Input: part model. Units: mm. Frame: model coordinates. A direction names the side the tool comes from. Give positions to 0.01 mm unless a question says otherwise; leave off trailing zeros. Loops run counter-clockwise (first coordinate to the right, second up) from the corner with the lowest first, then second, coordinate; pieces in that order, holes last. Notation, with made-up numbers: M 46,7 L 84,7 A15 cw 84,24 Z; hole C 42,84.25 d1. An arc over 180 degrees is marked long. One line per item, written item: value. Start each with the question number.
(1) Pin query (flat end, axial travel): P1, Ø5.5, axis at x = 6, y = 41.5, coming from the +Z side; P2, Ø1.5, axis at y = 27, z = 161.5, coming from the +X side; P3, Ø4, axis at x = -3, y = 46, coming from the -Z side. Return the tip coordinate at first contact, or that it passes through.
(2) Section D-D on z = -141. Output: boundary loops of the cut face in (x, y), plus the area to 3 significant figures.
(3) Pull-direction query (X, two-part tool) for faces 4 (the flat face through (-100.039, 54, -52)), 5 (the flat face through (-1, 38.1, 5)), 6 (the flat face through (3, 52.07, 68)), 7 (the flat face through (242.861, 22, -59)); classes: released by +X, released by -X, zero draft, split by the parting line, or undercut.
(4) Section A-A on x = 211.5. Output: boundary loops of the cut face in (y, z).
(5) Ray query, line 1 along Z through (x, y) = (94.5, 47); line 2 along Z through (x, y) = (-195, 30); line 3 along X through (y, z) = (31.5, 17). Return the intervals inside material, ascending. Write a range as from..to.
(6) Access query for faces 1 (the flat face through (-115, 24, -187.843)), 2 (the flat face through (-195, 22.86, -106)), 3 (the flat face through (-188.939, 22, 223)). Directions: +Z, -Z, +X, -X, +Y, -Y. A direction counts if a zero-diameter tool reaches every point of the face in a straight line with its end or side. Return the directions, or none.
(7) Section C-C on x = 35. Output: boundary loops of the cut face in (y, z).
(8) Section B-B on z = 120. Output: boundary loops of the cut face in (x, y).
```python
from build123d import *

# Parameters (mm, degrees)
SKETCH1_W                = 406.4
SKETCH1_H                = 406.4
SKETCH1_W_2              = 381
SKETCH1_H_2              = 381
BOSS_EXTRUDE2_DEPTH      = 38.1
SKETCH2_W                = 406.4
SKETCH2_H                = 406.4
BOSS_EXTRUDE3_DEPTH      = 5.08
CUT_EXTRUDE3_DEPTH       = 5.08
CUT_EXTRUDE4_DEPTH       = 446.859951222
CUT_EXTRUDE4_DEPTH_BACK  = 446.859951222
SKETCH6_R                = 5.08
CUT_EXTRUDE6_DEPTH       = 5.08
SKETCH8_W                = 457.2
SKETCH8_H                = 43.18
BOSS_EXTRUDE4_DEPTH      = 12.7
SKETCH9_R                = 5.08
CUT_EXTRUDE7_DEPTH       = 462.214953622
FILLET2_R                = 15.24
FILLET3_R                = 5.08
FILLET4_R                = 6.35
CUT_EXTRUDE8_DEPTH       = 473.102217157
CUT_EXTRUDE8_DEPTH_BACK  = 473.102217157
SKETCH10_W               = 25.4
SKETCH10_H               = 10.16
CUT_EXTRUDE9_DEPTH       = 316.013546928
CUT_EXTRUDE9_DEPTH_BACK  = 316.013546928
SKETCH11_W               = 10.16
SKETCH11_H               = 25.4
SKETCH13_W               = 38.1
SKETCH13_H               = 17.78
BOSS_EXTRUDE6_DEPTH      = 406.4
FILLET5_R                = 13.97
CUT_EXTRUDE10_DEPTH      = 475.059186858
CUT_EXTRUDE10_DEPTH_BACK = 101.6
SKETCH14_W               = 157.48
SKETCH14_H               = 20.829558228
SKETCH17_W               = 157.48
SKETCH17_H               = 21.78032637
CUT_EXTRUDE11_DEPTH      = 101.6
BOSS_EXTRUDE7_START      = -12.7
SKETCH18_W               = 375.92
SKETCH18_H               = 43.18
BOSS_EXTRUDE7_DEPTH      = 12.7
SKETCH19_W               = 12.7
SKETCH19_H               = 43.18
BOSS_EXTRUDE8_DEPTH      = 38.1
SKETCH20_R               = 5.08
CUT_EXTRUDE12_DEPTH      = 413.381445795
SKETCH21_W               = 23.212308842
SKETCH21_H               = 297.780762004
BOSS_EXTRUDE10_DEPTH     = 5.08
SKETCH22_W               = 25.4
SKETCH22_H               = 12.7
CUT_EXTRUDE13_DEPTH      = 500.147895153
SKETCH23_W               = 25.4
SKETCH23_H               = 12.7
CUT_EXTRUDE14_DEPTH      = 342.010118149


with BuildPart() as part:
    # Sketch1 → Boss-Extrude2 (new body)
    with BuildSketch(Plane(origin=(0, 0, 0), x_dir=(1, 0, 0), z_dir=(0, 1, 0))):
        with Locations((1.560576536, -7.736690009)):
            Rectangle(SKETCH1_W, SKETCH1_H)
        with Locations((1.560576536, -7.736690009)):
            Rectangle(SKETCH1_W_2, SKETCH1_H_2, mode=Mode.SUBTRACT)
    extrude(amount=BOSS_EXTRUDE2_DEPTH)

    # Sketch2 → Boss-Extrude3 (add)
    with BuildSketch(Plane(origin=(0, 38.1, 0), x_dir=(1, 0, 0), z_dir=(0, 1, 0))):
        with Locations((1.560576536, -7.736690009)):
            Rectangle(SKETCH2_W, SKETCH2_H)
    extrude(amount=BOSS_EXTRUDE3_DEPTH)

    # Sketch5 → Cut-Extrude3 (cut)
    with BuildSketch(Plane(origin=(0, 0, 198.236690009), x_dir=(-1, 0, 0), z_dir=(0, 0, -1))):
        Polygon((-115.860576536, 8.577585816), (-106.791199814, 13.813792908), (-106.791199814, 24.286207092), (-115.860576536, 29.522414184), (-124.929953259, 24.286207092), (-124.929953259, 13.813792908), align=None)
        Polygon((112.739423464, 29.522414184), (103.670046741, 24.286207092), (103.670046741, 13.813792908), (112.739423464, 8.577585816), (121.808800186, 13.813792908), (121.808800186, 24.286207092), align=None)
    extrude(amount=-CUT_EXTRUDE3_DEPTH, mode=Mode.SUBTRACT)

    # Sketch6 → Cut-Extrude4 (cut, two sides: drawn at the far end of the back side and taken through both)
    with BuildSketch(Plane(origin=(0, 0, 198.236690009), x_dir=(-1, 0, 0), z_dir=(0, 0, -1)).offset(-CUT_EXTRUDE4_DEPTH_BACK)):
        with Locations((-115.860576536, 19.05)):
            Circle(SKETCH6_R)
        with Locations((112.739423464, 19.05)):
            Circle(SKETCH6_R)
    extrude(amount=CUT_EXTRUDE4_DEPTH + CUT_EXTRUDE4_DEPTH_BACK, mode=Mode.SUBTRACT)

    # Sketch7 → Cut-Extrude6 (cut)
    with BuildSketch(Plane.XY.offset(-182.763309991)):
        Polygon((-112.739423464, 29.522414184), (-121.808800186, 24.286207092), (-121.808800186, 13.813792908), (-112.739423464, 8.577585816), (-103.670046741, 13.813792908), (-103.670046741, 24.286207092), align=None)
        Polygon((115.860576536, 29.522414184), (106.791199814, 24.286207092), (106.791199814, 13.813792908), (115.860576536, 8.577585816), (124.929953259, 13.813792908), (124.929953259, 24.286207092), align=None)
    extrude(amount=-CUT_EXTRUDE6_DEPTH, mode=Mode.SUBTRACT)

    # Sketch8 → Boss-Extrude4 (add)
    with BuildSketch(Plane.ZY.offset(201.639423464)):
        with Locations((7.736690009, 21.59)):
            Rectangle(SKETCH8_W, SKETCH8_H)
    extrude(amount=-BOSS_EXTRUDE4_DEPTH)

    # Sketch9 → Cut-Extrude7 (cut, through all)
    with BuildSketch(Plane(origin=(-188.939423464, 0, 0), x_dir=(0, 0, -1), z_dir=(1, 0, 0))):
        with Locations((208.163309991, 30.48)):
            Circle(SKETCH9_R)
        with Locations((-223.636690009, 30.48)):
            Circle(SKETCH9_R)
        with Locations((-223.636690009, 12.7)):
            Circle(SKETCH9_R)
        with Locations((208.163309991, 12.7)):
            Circle(SKETCH9_R)
    extrude(amount=-CUT_EXTRUDE7_DEPTH, mode=Mode.SUBTRACT)

    # Fillet2
    fillet2_edges = [part.edges().sort_by_distance(p)[0] for p in [
        (204.760576536, 21.59, 210.936690009),
        (204.760576536, 21.59, -195.463309991),
    ]]
    fillet(fillet2_edges, radius=FILLET2_R)

    # Fillet3
    fillet3_edges = [part.edges().sort_by_distance(p)[0] for p in [
        (-188.939423464, 21.59, -195.463309991),
        (-188.939423464, 21.59, 210.936690009),
    ]]
    fillet(fillet3_edges, radius=FILLET3_R)

    # Fillet4
    fillet4_edges = [part.edges().sort_by_distance(p)[0] for p in [
        (-195.289423464, 43.18, -220.863309991),
        (-195.289423464, 0, 236.336690009),
        (-201.639423464, 21.59, -220.863309991),
        (-201.639423464, 21.59, 236.336690009),
        (-188.939423464, 21.59, -220.863309991),
        (-195.289423464, 0, -220.863309991),
        (-188.939423464, 21.59, 236.336690009),
        (-195.289423464, 43.18, 236.336690009),
    ]]
    fillet(fillet4_edges, radius=FILLET4_R - 0.0001)  # a hair under: the kernel refuses the full size

    # Sketch10 → Cut-Extrude8 (cut, two sides: drawn at the far end of the back side and taken through both)
    with BuildSketch(Plane(origin=(204.760576536, 0, 0), x_dir=(0, 0, -1), z_dir=(1, 0, 0)).offset(-CUT_EXTRUDE8_DEPTH_BACK)):
        with Locations((-122.036690009, 17.78)):
            Rectangle(SKETCH10_W, SKETCH10_H)
        with Locations((106.563309991, 17.78)):
            Rectangle(SKETCH10_W, SKETCH10_H)
    extrude(amount=CUT_EXTRUDE8_DEPTH + CUT_EXTRUDE8_DEPTH_BACK, mode=Mode.SUBTRACT)

    # Sketch11 → Cut-Extrude9 (cut, two sides: drawn at the far end of the back side and taken through both)
    with BuildSketch(Plane(origin=(0, 38.1, 0), x_dir=(-1, 0, 0), z_dir=(0, -1, 0)).offset(-CUT_EXTRUDE9_DEPTH_BACK)):
        with Locations((-174.280576536, -122.036690009)):
            Rectangle(SKETCH11_W, SKETCH11_H)
        with Locations((171.159423464, -122.036690009)):
            Rectangle(SKETCH11_W, SKETCH11_H)
        with Locations((-174.280576536, 106.563309991)):
            Rectangle(SKETCH11_W, SKETCH11_H)
        with Locations((171.159423464, 106.563309991)):
            Rectangle(SKETCH11_W, SKETCH11_H)
    extrude(amount=CUT_EXTRUDE9_DEPTH + CUT_EXTRUDE9_DEPTH_BACK, mode=Mode.SUBTRACT)

    # Sketch13 → Boss-Extrude6 (add, through all)
    # profile 1 of 2: a face of its own
    with BuildSketch(Plane(origin=(204.760576536, 0, 0), x_dir=(0, 0, -1), z_dir=(1, 0, 0))):
        Polygon((-86.476690009, 60.96), (-86.476690009, 43.18), (-78.856690009, 43.18), (-78.856690009, 47.73825334), (-78.856690009, 52.07), (-55.996690009, 52.07), (-55.996690009, 48.121507739), (-55.996690009, 43.18), (-48.376690009, 43.18), (-48.376690009, 60.96), align=None)
    # profile 2 of 2: a face of its own
    with BuildSketch(Plane(origin=(204.760576536, 0, 0), x_dir=(0, 0, -1), z_dir=(1, 0, 0))):
        with Locations((51.953309991, 52.07)):
            Rectangle(SKETCH13_W, SKETCH13_H)
        Polygon((38.583459735, 43.205405435), (38.583459735, 47.763658775), (38.583459735, 52.07), (63.41669047, 52.07), (63.41669047, 47.763658775), (63.41669047, 43.205405435), align=None, mode=Mode.SUBTRACT)
    extrude(amount=-BOSS_EXTRUDE6_DEPTH)

    # Fillet5
    fillet5_edges = [part.edges().sort_by_distance(p)[0] for p in [
        (1.560576536, 60.96, 86.476690009),
        (1.560576536, 60.96, 48.376690009),
        (1.560576536, 60.96, -32.903309991),
        (1.560576536, 60.96, -71.003309991),
    ]]
    fillet(fillet5_edges, radius=FILLET5_R)

    # Sketch14 → Cut-Extrude10 (cut, two sides: drawn at the far end of the back side and taken through both)
    with BuildSketch(Plane.ZY.offset(201.639423464).offset(-CUT_EXTRUDE10_DEPTH_BACK)):
        with Locations((7.736690009, 53.594779114)):
            Rectangle(SKETCH14_W, SKETCH14_H)
    extrude(amount=CUT_EXTRUDE10_DEPTH + CUT_EXTRUDE10_DEPTH_BACK, mode=Mode.SUBTRACT)

    # Sketch17 → Cut-Extrude11 (cut)
    with BuildSketch(Plane(origin=(204.760576536, 0, 0), x_dir=(0, 0, -1), z_dir=(1, 0, 0))):
        with Locations((-7.736690009, 54.070163185)):
            Rectangle(SKETCH17_W, SKETCH17_H)
    extrude(amount=-CUT_EXTRUDE11_DEPTH, mode=Mode.SUBTRACT)

    # Sketch18 → Boss-Extrude7 (add)
    with BuildSketch(Plane(origin=(204.760576536, 0, 0), x_dir=(0, 0, -1), z_dir=(1, 0, 0)).offset(BOSS_EXTRUDE7_START)):
        with Locations((-7.736690009, 21.59)):
            Rectangle(SKETCH18_W, SKETCH18_H)
    extrude(amount=BOSS_EXTRUDE7_DEPTH)

    # Sketch19 → Boss-Extrude8 (add)
    with BuildSketch(Plane(origin=(204.760576536, 0, 0), x_dir=(0, 0, -1), z_dir=(1, 0, 0))):
        with Locations((84.973309991, 21.59)):
            Rectangle(SKETCH19_W, SKETCH19_H)
        with Locations((-100.446690009, 21.59)):
            Rectangle(SKETCH19_W, SKETCH19_H)
        with Locations((59.573309991, 21.59)):
            Rectangle(SKETCH19_W, SKETCH19_H)
        with Locations((-75.046690009, 21.59)):
            Rectangle(SKETCH19_W, SKETCH19_H)
    extrude(amount=BOSS_EXTRUDE8_DEPTH)

    # Sketch20 → Cut-Extrude12 (cut, through all)
    with BuildSketch(Plane.XY.offset(106.796690009)):
        with Locations((223.810576536, 21.59)):
            Circle(SKETCH20_R)
    extrude(amount=-CUT_EXTRUDE12_DEPTH, mode=Mode.SUBTRACT)

    # Sketch21 → Boss-Extrude10 (add)
    with BuildSketch(Plane.XZ.offset(-38.1)):
        with Locations((-170.393564794, 16.358404722)):
            Rectangle(SKETCH21_W, SKETCH21_H)
    extrude(amount=-BOSS_EXTRUDE10_DEPTH)

    # Sketch22 → Cut-Extrude13 (cut, through all)
    with BuildSketch(Plane(origin=(0, 0, -195.463309991), x_dir=(-1, 0, 0), z_dir=(0, 0, -1))):
        with Locations((-3.365108494, 17.400361313)):
            Rectangle(SKETCH22_W, SKETCH22_H)
    extrude(amount=-CUT_EXTRUDE13_DEPTH, mode=Mode.SUBTRACT)

    # Sketch23 → Cut-Extrude14 (cut, through all)
    with BuildSketch(Plane(origin=(0, 38.1, 0), x_dir=(-1, 0, 0), z_dir=(0, -1, 0))):
        with Locations((-3.365108494, -179.186690009)):
            Rectangle(SKETCH23_W, SKETCH23_H)
        with Locations((-3.365108494, 163.713309991)):
            Rectangle(SKETCH23_W, SKETCH23_H)
    extrude(amount=-CUT_EXTRUDE14_DEPTH, mode=Mode.SUBTRACT)


solid = part.part
```
Output values:
1. P1: stops at z = 210.94
1. P2: stops at x = 204.76
1. P3: stops at z = -71
2. outline: M -201.64,0 L -188.94,0 L -188.94,38.1 L 192.06,38.1 L 192.06,0 L 204.76,0 L 204.76,43.18 L -201.64,43.18 Z
2. area: 3,030 mm²
3. face 4: released by -X
3. face 5: undercut
3. face 6: zero draft
3. face 7: released by +X
4. outline: M 0,-91.32 L 43.18,-91.32 L 43.18,-78.62 L 0,-78.62 Z; M 0,-65.92 L 43.18,-65.92 L 43.18,-53.22 L 0,-53.22 Z; M 0,68.7 L 43.18,68.7 L 43.18,81.4 L 0,81.4 Z; M 0,94.1 L 43.18,94.1 L 43.18,106.8 L 0,106.8 Z
5. line 1: z = -71..-63.42, -38.58..-32.9, 48.38..56, 78.86..86.48
5. line 2: z = -220.86..-213.22, -203.11..218.58, 228.69..236.33
5. line 3: x = -201.64..-188.94, 192.06..204.76
6. face 1: none
6. face 2: -X
6. face 3: +Z, +X, +Y, -Y
7. outline: M 0,-195.46 L 43.18,-195.46 L 43.18,-71 L 46.99,-71 A13.97 ccw 60.96,-57.03 L 60.96,-46.87 A13.97 ccw 46.99,-32.9 L 43.18,-32.9 L 43.18,48.38 L 46.99,48.38 A13.97 ccw 60.96,62.35 L 60.96,72.51 A13.97 ccw 46.99,86.48 L 43.18,86.48 L 43.18,210.94 L 0,210.94 L 0,198.24 L 38.1,198.24 L 38.1,-182.76 L 0,-182.76 Z; hole M 43.18,56 L 52.07,56 L 52.07,78.86 L 43.18,78.86 Z; hole M 43.21,-63.42 L 52.07,-63.42 L 52.07,-38.58 L 43.21,-38.58 Z
8. outline: M -201.64,0 L -188.94,0 L -188.94,12.7 L -201.64,12.7 Z; M -201.64,22.86 L -188.94,22.86 L -188.94,38.1 L 169.2,38.1 L 169.2,43.18 L -201.64,43.18 Z; M 179.36,38.1 L 192.06,38.1 L 192.06,0 L 204.76,0 L 204.76,43.18 L 179.36,43.18 Z
